Could you check a few things on this model? Use its own coordinates, in mm. A direction names the side the tool comes from. Coordinates: 2 decimals unless noted, no trailing zeros. Write each loop counter-clockwise with the first axis right and the second up, starting at its lowest first coordinate (ties: lowest second). Pieces come first, ordered by that corner, then holes.
Item 1: Thinking about a two-plate mould opening in Y: for faces 1 (the flat face through (-3, 3, -6.35)), 2 (the flat face through (-3, 7, 0)), 3 (the flat face through (-3, -6.35, -105)), which applies, +Y half, -Y half, draft (parallel to the pull), parting line (faces both ways), or undercut?
Item 2: I want a section at D-D on z = -10.5. Please give me the cut outline in (x, y).
Item 3: I want a section at A-A on y = -4. Please give me the cut outline in (x, z).
Item 4: I want a section at C-C on y = 10.5. Please give me the cut outline in (x, z).
Item 5: Which directions (+Z, -Z, +X, -X, +Y, -Y) give clear straight access to the entire face, cutting with the end or side of a thin tool? Please do faces 4 (the flat face through (-3, 0, -60)), 5 (the flat face through (-3, -3, -12.7)), 6 (the flat face through (-3, 4.762, -118)), 7 (the flat face through (-3, 0, -114)).
Item 6: If I drill on probe 1 along Y at (x, z) = (-5.25, -59); probe 2 along Z at (x, y) = (-1.75, 2.5); probe 3 along Y at (x, z) = (-1.5, -6), over which ranges is the centre line in solid material (lowest first)?
Item 7: For P1, Ø1.9, axis at x = -2, z = -3.5, coming from the -Y side; P2, Ø1.5, axis at x = -2.5, y = -2.5, coming from the +Z side; P3, Ø1, axis at x = -4.5, y = 3, coming from the -Z side, each with a flat end and sliding along its axis, tell me the tip position at first contact or that it passes through.
Autodesk Inventor part; units mm, degrees
ref_plane "YZ Plane" through (0, 0, 0) normal (1, 0, 0) x (0, 1, 0)
ref_plane "XZ Plane" through (0, 0, 0) normal (0, 1, 0) x (-1, 0, 0)
ref_plane "XY Plane" through (0, 0, 0) normal (0, 0, 1) x (1, 0, 0)
sketch "Sketch1" plane through (0, 0, 0) normal (0, 1, 0) x (-1, 0, 0)
  line L0 (0, 0) -> (6.35, 0)
  line L1 (6.35, 0) -> (6.35, -120.65)
  line L2 (6.35, -120.65) -> (0, -120.65)
  line L3 (0, -120.65) -> (0, 0)
  dimension "d0" = 120.65
  dimension "d1" = 6.35
extrude "Extrusion1" add sketch "Sketch1" along normal blind 12.7
sketch "Sketch2" plane through (0, 0, 0) normal (0, -1, 0) x (1, 0, 0)
  line L0 (0, 0) -> (0, -120.65)
  line L1 (-6.35, -120.65) -> (-6.35, 0)
  line L2 (0, -12.7) -> (-6.35, -12.7)
  line L3 (-6.35, -12.7) -> (-6.35, -19.05)
  line L4 (-6.35, -19.05) -> (0, -19.05)
  line L5 (0, -19.05) -> (0, -12.7)
  line L6 (0, -101.6) -> (-6.35, -101.6)
  line L7 (-6.35, -101.6) -> (-6.35, -107.95)
  line L8 (-6.35, -107.95) -> (0, -107.95)
  line L9 (0, -107.95) -> (0, -101.6)
  line L10 (-6.35, -120.65) -> (0, -120.65)
  line L11 (0, 0) -> (-6.35, 0)
  dimension "d4" = 6.35
  dimension "d5" = 12.7
  dimension "d6" = 12.7
  dimension "d7" = 6.35
extrude "Extrusion2" add sketch "Sketch2" along normal blind 6.35 contours L0 L4 L1 L2 | L0 L8 L1 L6
sketch "Sketch3" plane through (0, 0, -120.65) normal (1, 0, 0) x (0, 0, -1)
  line L0 (-120.65, 0) -> (-120.65, 12.7)
  line L1 (-120.65, 4.7625) -> (-114.3, 4.7625)
  line L2 (-114.3, 4.7625) -> (-114.3, 1.5875)
  line L3 (-114.3, 1.5875) -> (-120.65, 1.5875)
  line L4 (-120.65, 1.5875) -> (-120.65, 4.7625)
  line L5 (0, 0) -> (0, 12.7)
  line L6 (0, 4.7625) -> (-6.35, 4.7625)
  line L7 (-6.35, 4.7625) -> (-6.35, 1.5875)
  line L8 (-6.35, 1.5875) -> (0, 1.5875)
  line L9 (0, 1.5875) -> (0, 4.7625)
  line L10 (-107.95, 0) -> (-120.65, 0)
  dimension "d10" = 6.35
  dimension "d11" = 3.175
  dimension "d12" = 1.5875
  dimension "d13" = 6.35
extrude "Extrusion3" cut sketch "Sketch3" against normal blind 6.35
sketch "Sketch4" plane through (0, 12.7, 0) normal (1, 0, 0) x (0, 0, -1)
  line L0 (0, -7.9375) -> (0, 0)
  line L1 (120.65, -7.9375) -> (120.65, 0)
  arc A0 (0, 0) -> (120.65, 0) centre (60.325, 555.5343) ccw
  line L2 (120.65, 0) -> (0, 0)
  line L3 (0, 0) -> (120.65, 0)
  point P0 (0, -12.7)
  dimension "d16" = 558.8
extrude "Extrusion4" cut sketch "Sketch4" against normal blind 6.35
fillet "Fillet1" radius 3.175 2 edges at (-3.175, 12.7, 0) (-3.175, 12.7, -120.65)
properties part number "MonsterHolderSupport2"
Response values:
1. face 1: undercut
1. face 2: draft
1. face 3: -Y half
2. outline: (-6.35, 0) - (0, 0) - (0, 11.66) - (-6.35, 11.66) - close
3. outline: (-6.35, -107.95) - (0, -107.95) - (0, -101.6) - (-6.35, -101.6) - close; (-6.35, -19.05) - (0, -19.05) - (0, -12.7) - (-6.35, -12.7) - close
4. outline: (-6.35, -120.36) - (0, -120.36) - (0, -94.82) - (-6.35, -94.82) - close; (-6.35, -25.83) - (0, -25.83) - (0, -0.29) - (-6.35, -0.29) - close
5. face 4: +X, -X, -Y
5. face 5: +Z, +X, -X, -Y
5. face 6: -Z, +X, -X
5. face 7: -Z, +X, -X, -Y
6. probe 1: y = 0 to 9.44
6. probe 2: z = -114.3 to -6.35
6. probe 3: y = 0 to 1.59, 4.76 to 12.08
7. P1: stops at y = 0
7. P2: stops at z = -12.7
7. P3: stops at z = -114.3
